Read the model definition and answer for the solid it produces. Units are mm, in the model's axes. A direction names the side the tool comes from. Coordinates: 2 decimals unless noted, no trailing zeros. Loops run counter-clockwise (first coordinate to the right, second up) from the corner with the lowest first, then second, coordinate; pieces in that order, holes last.
Q1. Flat-ended cylindrical pins translate along their axes: P1, Ø6, axis at y = 4.5, z = 38.5, coming from the -X side; P2, Ø14, axis at y = 12.79, z = 0, coming from the +X side; P3, Ø13, axis at y = 11, z = -2, coming from the -X side; P4, Ø10, axis at y = 3.5, z = -30, coming from the -X side. Find the tip coordinate at first contact, or state that the pin passes through.
Q2. Section B-B (x = -95) is taken. Give the vertices of the cut face in (y, z).
Q3. Straight lines are drawn through the part: line 1 (X direction, y = -5, z = -102); line 2 (Z direction, x = 111, y = -5.5); line 3 (Y direction, x = 55.5, z = -47.5). For each, find the intervals that lie inside material, in ascending order.
Q4. The mould has two halves that part along Y. Classify faces 6 (the face through (0.089, 7.079, 8.057)), 7 (the face through (-0.1, 16.9, -1.7)), 8 (the face through (-2, -4, -134.62)): pulls with the +Y half, pulls with the -Y half, needs draft (parallel to the pull), parting line crosses it, or undercut.
Q5. Section A-A (z = 16) is taken. Give the vertices of the cut face in (x, y), then the cut area to 3 significant figures.
Q6. Which of the six approach directions +Z, -Z, +X, -X, +Y, -Y give full straight-line access (tool end or side, diameter ignored) to faces 1 (the face through (6.35, 8, 1)), 2 (the face through (-172.72, -4, -2)), 3 (the face through (172.72, -4, -2)), 4 (the face through (-6.35, 8, 1)), 5 (the face through (-2, -2.54, 2))?
from build123d import *

# Parameters (mm, degrees)
F0_W     = 304.8
F0_H     = 228.6
F1_DEPTH = 2.54
F0_W_2   = 345.44
F0_H_2   = 269.24
F2_DEPTH = 7.62
F3_R     = 4.445
F4_DEPTH = 6.35


with BuildPart() as f1:
    # F0 (on Front) → F1 (new body)
    with BuildSketch(Plane.XZ):
        Rectangle(F0_W, F0_H)
    extrude(amount=F1_DEPTH)

    # F0 (on Front) → F2 (join)
    with BuildSketch(Plane.XZ):
        Rectangle(F0_W_2, F0_H_2)
        Rectangle(F0_W, F0_H, mode=Mode.SUBTRACT)
    extrude(amount=F2_DEPTH)

    # F3 (on Right) → F4 (join, symmetric)
    with BuildSketch(Plane.YZ):
        with BuildLine():
            Line((13.962311, 6.886105), (0, 9.260906))
            Line((0, 9.260906), (0, -6.802539))
            Line((0, -6.802539), (12.691058, -6.984284))
            ThreePointArc((12.691058, -6.984284), (5.835232, 0.63752), (13.962311, 6.886105))
        make_face()
        with BuildLine():
            ThreePointArc((19.776078, 0), (18.128272, 4.50606), (13.962311, 6.886105))
            ThreePointArc((13.962311, 6.886105), (5.835232, 0.63752), (12.691058, -6.984284))
            ThreePointArc((12.691058, -6.984284), (17.694729, -4.974378), (19.776078, 0))
        make_face()
        with Locations((12.791078, 0)):
            Circle(F3_R, mode=Mode.SUBTRACT)
    extrude(amount=F4_DEPTH, both=True)


solid = f1.part
Numbers:
1. P1: passes through
1. P2: stops at x = 6.35
1. P3: stops at x = -6.35
1. P4: stops at x = -172.72
2. outline: (-7.62, -134.62) - (0, -134.62) - (0, 134.62) - (-7.62, 134.62) - (-7.62, 114.3) - (-2.54, 114.3) - (-2.54, -114.3) - (-7.62, -114.3) - close
3. line 1: x = -172.72 to -152.4, 152.4 to 172.72
3. line 2: z = -134.62 to -114.3, 114.3 to 134.62
3. line 3: y = -2.54 to 0
4. face 6: pulls with the +Y half
4. face 7: undercut
4. face 8: needs draft
5. outline: (-172.72, -7.62) - (-152.4, -7.62) - (-152.4, -2.54) - (152.4, -2.54) - (152.4, -7.62) - (172.72, -7.62) - (172.72, 0) - (-172.72, 0) - close
5. area: 1,080 mm2
6. face 1: +Z, -Z, +X, +Y
6. face 2: +Z, -Z, -X, +Y, -Y
6. face 3: +Z, -Z, +X, +Y, -Y
6. face 4: +Z, -Z, -X, +Y
6. face 5: -Y
